Source: CAD feature listing. Evaluate the final solid. Frame: model axes, mm. Coordinates: 2 decimals unless noted, no trailing zeros. Loops run counter-clockwise (first coordinate to the right, second up) from the corner with the lowest first, then second, coordinate; pieces in that order, holes last. Notation, with made-up numbers: M -9,60 L 46,60 A27 cw 46,99 Z; hole C 82.25,-32.5 d2. An arc over 180 degrees is marked long. One line per question, with ' | ' between items. Start each with the question number.
1. Pin query (flat end, axial travel): P1, Ø3, axis at y = -4, z = 19, coming from the +X side; P2, Ø1.5, axis at x = 2, z = 35, coming from the -Y side; P3, Ø3.5, axis at x = 0, y = 0, coming from the -Z side. Return the tip coordinate at first contact, or that it passes through.
2. Section query D-D, the plane y = 5.25. Output: boundary loops of the cut face in (x, z), and give its area (3 significant figures).
3. Section query C-C, the plane z = 53. Output: boundary loops of the cut face in (x, y), and give its area (3 significant figures).
4. Ray query, probe 1 along X at (y, z) = (1, 61); probe 2 along Y at (x, z) = (0, 58.25); probe 3 along X at (y, z) = (-2.5, 61). Return the intervals inside material, ascending.
5. Section query A-A, the plane x = 0. Output: boundary loops of the cut face in (y, z), and give its area (3 significant figures).
Autodesk Fusion 360 part; units mm, degrees
sketch "スケッチ1" plane through (0, 0, 0) normal (0, 0, 1) x (1, 0, 0)
  circle A0 centre (0, 0) radius 6
  dimension "d1" = 12
extrude "押し出し1" add sketch "スケッチ1" along normal blind 69
cylinder "円柱プリミティブ1" cut diameter 6 height -15 placed x (1, 0, 0) y (0, 1, 0) z (0, 0, 1) at (0, 0, 69)
thread "ねじ1" thread offset 0 thread length 10
cylinder "円柱プリミティブ2" cut diameter 6 height -15 placed x (0, 1, 0) y (1, 0, 0) z (0, 0, -1) at (0, 0, 0)
thread "ねじ2" thread offset 0 thread length 10
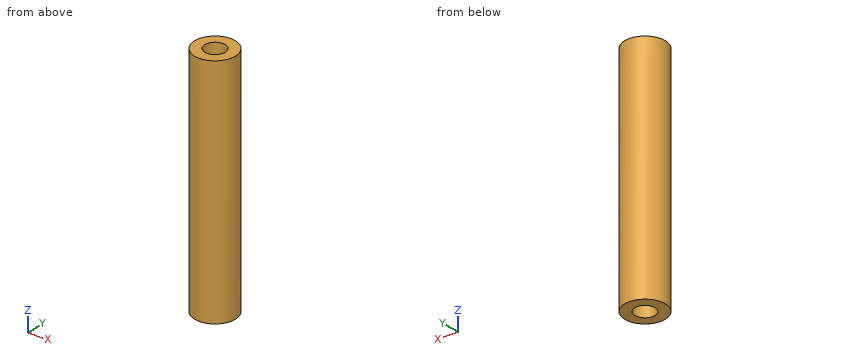
Taken from the geometry:
1) P1: x = 5.45 | P2: y = -5.87 | P3: z = 15
2) outline: M -2.9,0 L 2.9,0 L 2.9,69 L -2.9,69 Z | area: 401 mm^2
3) outline: C 0,0 d12 | area: 113 mm^2
4) probe 1: -5.92 to -2.83, 2.83 to 5.92 | probe 2: -6 to -3, 3 to 6 | probe 3: -5.45 to -1.66, 1.66 to 5.45
5) outline: M -6,0 L -3,0 L -3,15 L 3,15 L 3,0 L 6,0 L 6,69 L 3,69 L 3,54 L -3,54 L -3,69 L -6,69 Z | area: 648 mm^2
